Source: CAD feature listing. Evaluate the final solid. Frame: model axes, mm. A direction names the side the tool comes from. Round coordinates to 2 decimals unless told otherwise and drop trailing zeros. Write each loop counter-clockwise with the first axis right and the second up, starting at its lowest first coordinate (ties: lowest second). Pieces come first, ordered by that corner, then holes. Notation, with made-up numbers: M 71,-39.5 L 129,-39.5 A23 cw 129,-15.5 Z; hole C 77,53 d1. An arc over 180 degrees is marked long. Use a Markdown table: item, result.
```python
from build123d import *

# Parameters (mm, degrees)
SCHIZZO1_W                    = 485
SCHIZZO1_H                    = 270
ESTRUSIONE_ESTRUSIONE1_DEPTH  = 10
FORO_PER_VITE_M8_1_OUTLINE_R  = 4.5
FORO_PER_VITE_M8_1_DEPTH      = 10
TAGLIO_ESTRUSIONE1_DEPTH      = 13
TAGLIO_ESTRUSIONE1_DEPTH_BACK = 13
SCHIZZO5_W                    = 91.448812178
SCHIZZO5_H                    = 10
SCHIZZO6_R                    = 2.25
TAGLIO_ESTRUSIONE2_DEPTH      = 10
SCHIZZO7_R                    = 1.75
TAGLIO_ESTRUSIONE3_DEPTH      = 15
SCHIZZO8_R                    = 2.25
TAGLIO_ESTRUSIONE4_DEPTH      = 42.3
SCHIZZO9_W                    = 30
SCHIZZO9_H                    = 15
TAGLIO_ESTRUSIONE5_DEPTH      = 10
SCHIZZO10_R                   = 2.25
TAGLIO_ESTRUSIONE6_DEPTH      = 10


# Read off the part's stored shape, not the designer's step: Foro per Vite M8-1
with BuildPart() as part:
    # Schizzo1 → Estrusione-Estrusione1 (new body)
    with BuildSketch(Plane(origin=(0, 0, 0), x_dir=(1, 0, 0), z_dir=(0, 1, 0))):
        with Locations((-242.5, 135)):
            Rectangle(SCHIZZO1_W, SCHIZZO1_H)
    extrude(amount=ESTRUSIONE_ESTRUSIONE1_DEPTH)

    # Foro per Vite M8-1 outline → Foro per Vite M8-1 (cut)
    with BuildSketch(Plane(origin=(0, 0, 0), x_dir=(1, 0, 0), z_dir=(0, 1, 0))):
        with Locations((-205, 250)):
            Circle(FORO_PER_VITE_M8_1_OUTLINE_R)
        with Locations((-465, 20)):
            Circle(FORO_PER_VITE_M8_1_OUTLINE_R)
        with Locations((-205, 20)):
            Circle(FORO_PER_VITE_M8_1_OUTLINE_R)
        with Locations((-465, 250)):
            Circle(FORO_PER_VITE_M8_1_OUTLINE_R)
    extrude(amount=FORO_PER_VITE_M8_1_DEPTH, mode=Mode.SUBTRACT)

    # Schizzo5 → Taglio-Estrusione1 (cut, two sides: drawn at the far end of the back side and taken through both)
    with BuildSketch(Plane(origin=(-128.208113313, 0, -287.960137213), x_dir=(0.9135454576425992, 0, -0.4067366430758042), z_dir=(0.4067366430758042, 0, 0.9135454576425992)).offset(-TAGLIO_ESTRUSIONE1_DEPTH_BACK)):
        with Locations((-228.551173826, 5)):
            Rectangle(SCHIZZO5_W, SCHIZZO5_H)
    extrude(amount=TAGLIO_ESTRUSIONE1_DEPTH + TAGLIO_ESTRUSIONE1_DEPTH_BACK, mode=Mode.SUBTRACT)

    # Schizzo6 → Taglio-Estrusione2 (cut)
    with BuildSketch(Plane(origin=(0, 10, 0), x_dir=(1, 0, 0), z_dir=(0, 1, 0))):
        with Locations(Location((-48.207846429, 223.792153571, 0), (0, 0, 270))):
            Circle(SCHIZZO6_R)
        with Locations(Location((-215.792153571, 223.792153571, 0), (0, 0, 270))):
            Circle(SCHIZZO6_R)
        with Locations(Location((-215.792153571, 56.207846429, 0), (0, 0, 270))):
            Circle(SCHIZZO6_R)
        with Locations(Location((-48.207846429, 56.207846429, 0), (0, 0, 270))):
            Circle(SCHIZZO6_R)
    extrude(amount=-TAGLIO_ESTRUSIONE2_DEPTH, mode=Mode.SUBTRACT)

    # Schizzo7 → Taglio-Estrusione3 (cut)
    with BuildSketch(Plane(origin=(0, 10, 0), x_dir=(1, 0, 0), z_dir=(0, 1, 0))):
        with Locations(Location((-147.5, 155.5, 0), (0, 0, 270))):
            Circle(SCHIZZO7_R)
        with Locations(Location((-116.5, 155.5, 0), (0, 0, 270))):
            Circle(SCHIZZO7_R)
        with Locations(Location((-116.5, 124.5, 0), (0, 0, 270))):
            Circle(SCHIZZO7_R)
        with Locations(Location((-147.5, 124.5, 0), (0, 0, 270))):
            Circle(SCHIZZO7_R)
    extrude(amount=-TAGLIO_ESTRUSIONE3_DEPTH, mode=Mode.SUBTRACT)

    # Schizzo8 → Taglio-Estrusione4 (cut)
    with BuildSketch(Plane(origin=(0, 10, 0), x_dir=(1, 0, 0), z_dir=(0, 1, 0))):
        with Locations(Location((-327.299756602, 243.651595895, 0), (0, 0, 270))):
            Circle(SCHIZZO8_R)
        with Locations(Location((-379.645911325, 220.345586247, 0), (0, 0, 270))):
            Circle(SCHIZZO8_R)
    extrude(amount=-TAGLIO_ESTRUSIONE4_DEPTH, mode=Mode.SUBTRACT)

    # Schizzo9 → Taglio-Estrusione5 (cut)
    with BuildSketch(Plane(origin=(0, 10, 0), x_dir=(1, 0, 0), z_dir=(0, 1, 0))):
        with Locations((-15, 262.5)):
            Rectangle(SCHIZZO9_W, SCHIZZO9_H)
        with Locations((-15, 7.5)):
            Rectangle(SCHIZZO9_W, SCHIZZO9_H)
        with Locations((-391.074312, 262.5)):
            Rectangle(SCHIZZO9_W, SCHIZZO9_H)
    extrude(amount=-TAGLIO_ESTRUSIONE5_DEPTH, mode=Mode.SUBTRACT)

    # Schizzo10 → Taglio-Estrusione6 (cut)
    with BuildSketch(Plane(origin=(0, 10, 0), x_dir=(1, 0, 0), z_dir=(0, 1, 0))):
        with Locations(Location((-20, 35, 0), (0, 0, 270))):
            Circle(SCHIZZO10_R)
        with Locations(Location((-20, 235, 0), (0, 0, 270))):
            Circle(SCHIZZO10_R)
    extrude(amount=-TAGLIO_ESTRUSIONE6_DEPTH, mode=Mode.SUBTRACT)


solid = part.part
```
Q1. Section B-B on x = -314. Return loops of the section in (y, z).
Results are:
| item | result |
|---|---|
| outline | M 0,-270 L 10,-270 L 10,-219.47 L 0,-219.47 Z; M 0,-191.01 L 10,-191.01 L 10,0 L 0,0 Z |
Q2. Mould query, pull axis Z, two halves, no side actions, for faces 4 (the flat face through (-261, 5, 0)), 5 (the cylindrical face through (-200.84, 4.93, -248.28)), 6 (the flat face through (-332.297, 5.07, -182.864)), 7 (the flat face through (-485, 5, -133)). Classes: +Z half, -Z half, draft (parallel to the pull), parting line (faces both ways), or undercut.
Results are:
| item | result |
|---|---|
| face 4 | +Z half |
| face 5 | undercut |
| face 6 | undercut |
| face 7 | draft |
Q3. Section A-A on z = -20. Return loops of the section in (x, y).
Results are:
| item | result |
|---|---|
| outline | M -485,0 L -469.5,0 L -469.5,10 L -485,10 Z; M -460.5,0 L -209.5,0 L -209.5,10 L -460.5,10 Z; M -200.5,0 L 0,0 L 0,10 L -200.5,10 Z |
Q4. Reachability of faces 1 (the flat face through (-406.074, 5, -262)), 2 (the flat face through (-30, 5, -262)), 3 (the flat face through (-15, 5, -15)) from +Z, -Z, +X, -X, +Y, -Y: full face, straight path, thin tool, end or side. Return the list, or none.
Results are:
| item | result |
|---|---|
| face 1 | -Z, +Y, -Y |
| face 2 | -Z, +X, +Y, -Y |
| face 3 | +Z, +X, +Y, -Y |
Q5. Section C-C on y = 5.75. Give the number of separate pieces and of enclosed holes in the cut face, plus the area to 3 significant figures.
Results are:
| item | result |
|---|---|
| separate pieces | 1 |
| enclosed holes | 17 |
| area | 127,000 mm^2 |
Q6. Line query: L1, parallel to Z at x = -116.5, y = 5.75; L2, parallel to X at y = 3.5, z = -155.5; L3, parallel to Z at x = -465, y = 5. Output: solid intervals per line, ascending.
Results are:
| item | result |
|---|---|
| L1 | -270 to -157.25, -153.75 to -126.25, -122.75 to 0 |
| L2 | -485 to -149.25, -145.75 to -118.25, -114.75 to 0 |
| L3 | -270 to -254.5, -245.5 to -24.5, -15.5 to 0 |
Q7. First-contact query: pin 1 Ø14.5 at (x, z) = (-465, -20) entering from -Y; pin 2 Ø5 at (y, z) = (5.5, -261) entering from +X; pin 3 Ø2 at (x, z) = (-147.5, -124.5) entering from +Y. Flat tips, straight axial feed; report the tip coordinate or a pass-through.
Results are:
| item | result |
|---|---|
| pin 1 | y = 0 |
| pin 2 | x = -30 |
| pin 3 | through |
